```python
from build123d import *

# Parameters (mm, degrees)
SKETCH_1_W          = 40
SKETCH_1_H          = 20
EXTRUDE_1_DEPTH     = 40
SKETCH_2_R          = 3
SKETCH_2_R_2        = 1.5
EXTRUDE_2_DEPTH     = 3.5
SKETCH_3_R          = 6
EXTRUDE_3_DEPTH     = 1
EXTRUDE_START       = 6
SKETCH_4_R          = 3
SKETCH_4_R_2        = 1
EXTRUDE_4_DEPTH     = 6
SKETCH_5_R          = 0.5
CUT_EXTRUDE_1_DEPTH = 10
CUT_EXTRUDE_START   = -10
SKETCH_6_R          = 0.5
CUT_EXTRUDE_2_DEPTH = 10


with BuildPart() as part:
    # 草图1 → 凸台-拉伸1 (new body)
    with BuildSketch(Plane.XY):
        Rectangle(SKETCH_1_W, SKETCH_1_H)
    extrude(amount=EXTRUDE_1_DEPTH)

    # 草图2 → 凸台-拉伸2 (add)
    with BuildSketch(Plane.XY.offset(40)):
        with Locations(Location((10, 0, 0), (0, 0, 180))):
            Circle(SKETCH_2_R)
        with Locations((10, 0)):
            Circle(SKETCH_2_R_2, mode=Mode.SUBTRACT)
    extrude(amount=EXTRUDE_2_DEPTH)

    # 草图3 → 凸台-拉伸3 (add)
    with BuildSketch(Plane(origin=(0, 0, 0), x_dir=(-1, 0, 0), z_dir=(0, 0, -1))):
        with Locations((-10, 0)):
            Circle(SKETCH_3_R)
    extrude(amount=EXTRUDE_3_DEPTH)

    # 草图4 → 凸台-拉伸4 (add)
    with BuildSketch(Plane(origin=(0, 0, -1), x_dir=(-1, 0, 0), z_dir=(0, 0, -1)).offset(EXTRUDE_START)):
        with Locations((-10, 0)):
            Circle(SKETCH_4_R)
        with Locations((-10, 0)):
            Circle(SKETCH_4_R_2, mode=Mode.SUBTRACT)
    extrude(amount=-EXTRUDE_4_DEPTH)

    # 草图5 → 切除-拉伸1 (cut)
    with BuildSketch(Plane.XY.offset(40)):
        with Locations((-18, 0)):
            Circle(SKETCH_5_R)
        with Locations((-11, 8)):
            Circle(SKETCH_5_R)
        with Locations((0, 9)):
            Circle(SKETCH_5_R)
        with Locations((-11, -8)):
            Circle(SKETCH_5_R)
        with Locations((0, -9)):
            Circle(SKETCH_5_R)
    extrude(amount=-CUT_EXTRUDE_1_DEPTH, mode=Mode.SUBTRACT)

    # 草图6 → 切除-拉伸2 (cut)
    with BuildSketch(Plane(origin=(0, 0, 0), x_dir=(-1, 0, 0), z_dir=(0, 0, -1)).offset(CUT_EXTRUDE_START)):
        with Locations(Location((18, 0, 0), (0, 0, 180))):
            Circle(SKETCH_6_R)
        with Locations(Location((11, -8, 0), (0, 0, 180))):
            Circle(SKETCH_6_R)
        with Locations(Location((0, -9, 0), (0, 0, 180))):
            Circle(SKETCH_6_R)
        with Locations(Location((11, 8, 0), (0, 0, 180))):
            Circle(SKETCH_6_R)
        with Locations(Location((0, 9, 0), (0, 0, 180))):
            Circle(SKETCH_6_R)
    extrude(amount=CUT_EXTRUDE_2_DEPTH, mode=Mode.SUBTRACT)


solid = part.part
```
Read the model definition and answer for the solid it produces. Units are mm, in the model's axes. A direction names the side the tool comes from. Give positions to 0.01 mm unless a question says otherwise; leave off trailing zeros. Order: outer loops, then holes, each group sorted by start corner. A loop starts at its lowest first (then second) coordinate and runs counter-clockwise, first axis right, second up.
(1) Find section B-B (y = -4.5). Give the vertices of the cut face in (x, z), plus the area to 3 significant figures.
(2) Given pin 1 (10 mm diameter, centred on x = -11, y = 8, fed in from -Z); pin 2 (0.8 mm diameter, centred on x = 0, y = 9, fed in from -Z); pin 3 (0.8 mm diameter, centred on x = 0, y = -9, fed in from +Z); pin 4 (2.5 mm diameter, centred on x = 10, y = 0, fed in from -Z), each flat-ended and moving along its own axis, determine where each tip first touches the part or whether it passes through.
(3) Find section A-A (x = 10). Give the vertices of the cut face in (y, z), plus the area to 4 significant figures.
(4) For faces 5 (the cylindrical face through (13, 0, 42)), 6 (the flat face through (13, -1, -1)), 7 (the flat face through (8.7, 1.3, 43.5)), determine the directions among +Z, -Z, +X, -X, +Y, -Y from which every point of the face is accessible in a straight line to the end or side of a thin tool.
(5) Straight lines are drawn through the part: L1, parallel to Y at x = -11, z = 1.5; L2, parallel to Y at x = -18, z = 5.75; L3, parallel to Z at x = 4.5, y = 8. For each, find the intervals that lie inside material, in ascending order.
(6) For a pull along Y with two mould halves and no side action, classify faces 1 (the flat face through (10, 0, 40)), 2 (the flat face through (20, 0, 20)), 3 (the flat face through (10, 0, -1)), 4 (the flat face through (0, -10, 20)) as released by +Y, released by -Y, zero draft, split by the parting line, or undercut.
(7) Find section C-C (x = 17.5). Give the vertices of the cut face in (y, z), plus the area to 3 significant figures.
Result sheet:
1. outline: (-20, 0) - (6.03, 0) - (6.03, -1) - (13.97, -1) - (13.97, 0) - (20, 0) - (20, 40) - (-20, 40) - close
1. area: 1,610 mm2
2. pin 1: stops at z = 0
2. pin 2: stops at z = 10
2. pin 3: stops at z = 30
2. pin 4: stops at z = -7
3. outline: (-10, 0) - (-6, 0) - (-6, -1) - (-3, -1) - (-3, -7) - (-1, -7) - (-1, -1) - (1, -1) - (1, -7) - (3, -7) - (3, -1) - (6, -1) - (6, 0) - (10, 0) - (10, 40) - (3, 40) - (3, 43.5) - (1.5, 43.5) - (1.5, 40) - (-1.5, 40) - (-1.5, 43.5) - (-3, 43.5) - (-3, 40) - (-10, 40) - close
3. area: 846.5 mm2
4. face 5: +Z
4. face 6: -Z
4. face 7: +Z, +X, -X, +Y, -Y
5. L1: y = -10 to -8.5, -7.5 to 7.5, 8.5 to 10
5. L2: y = -10 to -0.5, 0.5 to 10
5. L3: z = 0 to 40
6. face 1: undercut
6. face 2: zero draft
6. face 3: undercut
6. face 4: released by -Y
7. outline: (-10, 0) - (10, 0) - (10, 40) - (-10, 40) - close
7. area: 800 mm2
